Can you work these out from the model? Positions are in its coordinate system, mm. A direction names the side the tool comes from. Give positions to 0.01 mm unless a question says otherwise; leave off trailing zeros. Order: outer loops, then holes, each group sorted by start corner. A loop starts at its lowest first (then second) coordinate and runs counter-clockwise, first axis right, second up.
Item 1: I want a section at C-C, the plane y = -3.5. Write out the boundary of the cut face in (x, z).
Item 2: I'm going to push flat-ended pins straight in: pin 1 Ø3 at (x, y) = (7.5, 3.5) entering from +Z; pin 2 Ø1.5 at (x, y) = (3.5, 7.5) entering from -Z; pin 3 Ø1.5 at (x, z) = (2.5, 2.5) entering from +Y; pin 4 Ø1.5 at (y, z) = (-0.5, 4) entering from -X. Where does each tip first touch, or does it pass through?
Item 3: If we mould it in two halves opening along X, with no side actions, what happens to faces 1 (the cylindrical face through (-2.923, 6.391, 0.986)), 2 (the cylindrical face through (2.285, 3.584, 3.972)), 3 (the cylindrical face through (-3.77, -8.72, 0.99)), 4 (the flat face through (2.5, 2.5, 0))? For each: +X half, -X half, draft (parallel to the pull), parting line (faces both ways), or undercut.
Item 4: I want a section at D-D, the plane z = 1.75. Count the separate pieces of the cut face and the enclosed holes in it, then the cut area to 3 significant figures.
Item 5: I want a section at B-B, the plane y = 7.5. Write out the boundary of the cut face in (x, z), then the cut area to 3 significant figures.
Item 6: Which directions (+Z, -Z, +X, -X, +Y, -Y) give clear straight access to the entire face, cutting with the end or side of a thin tool? Please do faces 5 (the cylindrical face through (10, 3.2, 1)), 6 (the flat face through (5, 0, 2)).
Item 7: If I drill on line 1 along Y through (x, z) = (6.5, 1.9); line 2 along Z through (x, y) = (8.5, 4.75); line 3 along X through (y, z) = (-1.25, 4.7), over which ranges is the centre line in solid material (lowest first)?
Item 8: I want a section at A-A, the plane x = -7.75. Write out the boundary of the cut face in (y, z).
```python
from build123d import *

# Parameters (mm, degrees)
SKETCH5_R           = 10.5
SKETCH5_R_2         = 1.25
BOSS_EXTRUDE2_DEPTH = 2
SKETCH6_R           = 1.25
CUT_EXTRUDE2_DEPTH  = 2
SKETCH7_R           = 3
CUT_EXTRUDE3_DEPTH  = 1
SKETCH9_R           = 3
CUT_EXTRUDE5_DEPTH  = 5
SKETCH10_R          = 3
BOSS_EXTRUDE5_DEPTH = 2
SKETCH11_R          = 3.25
CUT_EXTRUDE6_DEPTH  = 2
SKETCH13_R          = 4.25
SKETCH13_R_2        = 3.25
BOSS_EXTRUDE6_DEPTH = 4


with BuildPart() as part:
    # Sketch5 → Boss-Extrude2 (new body)
    with BuildSketch(Plane.XY):
        Circle(SKETCH5_R)
        with Locations((0, 7.5)):
            Circle(SKETCH5_R_2, mode=Mode.SUBTRACT)
        with Locations((-3.5, 7.5)):
            Circle(SKETCH5_R_2, mode=Mode.SUBTRACT)
        with Locations((3.5, 7.5)):
            Circle(SKETCH5_R_2, mode=Mode.SUBTRACT)
        with Locations((-7.5, 0)):
            Circle(SKETCH5_R_2, mode=Mode.SUBTRACT)
        with Locations((-7.5, 3.5)):
            Circle(SKETCH5_R_2, mode=Mode.SUBTRACT)
        with Locations((-7.5, -3.5)):
            Circle(SKETCH5_R_2, mode=Mode.SUBTRACT)
        with Locations((0, -7.5)):
            Circle(SKETCH5_R_2, mode=Mode.SUBTRACT)
        with Locations((-3.5, -7.5)):
            Circle(SKETCH5_R_2, mode=Mode.SUBTRACT)
        with Locations((3.499264905, -7.428270452)):
            Circle(SKETCH5_R_2, mode=Mode.SUBTRACT)
        with Locations((7.5, 0)):
            Circle(SKETCH5_R_2, mode=Mode.SUBTRACT)
        with Locations((7.5, 3.5)):
            Circle(SKETCH5_R_2, mode=Mode.SUBTRACT)
        with Locations((7.5, -3.5)):
            Circle(SKETCH5_R_2, mode=Mode.SUBTRACT)
    extrude(amount=BOSS_EXTRUDE2_DEPTH)

    # Sketch6 → Cut-Extrude2 (cut)
    with BuildSketch(Plane(origin=(0, 0, 0), x_dir=(-1, 0, 0), z_dir=(0, 0, -1))):
        Circle(SKETCH6_R)
    extrude(amount=-CUT_EXTRUDE2_DEPTH, mode=Mode.SUBTRACT)

    # Sketch7 → Cut-Extrude3 (cut)
    with BuildSketch(Plane(origin=(0, 0, 0), x_dir=(-1, 0, 0), z_dir=(0, 0, -1))):
        Circle(SKETCH7_R)
    extrude(amount=-CUT_EXTRUDE3_DEPTH, mode=Mode.SUBTRACT)

    # Sketch9 → Cut-Extrude5 (cut)
    with BuildSketch(Plane(origin=(0, 0, 0), x_dir=(-1, 0, 0), z_dir=(0, 0, -1))):
        Circle(SKETCH9_R)
    extrude(amount=-CUT_EXTRUDE5_DEPTH, mode=Mode.SUBTRACT)

    # Sketch10 → Boss-Extrude5 (add)
    with BuildSketch(Plane(origin=(0, 0, 0), x_dir=(-1, 0, 0), z_dir=(0, 0, -1))):
        Circle(SKETCH10_R)
    extrude(amount=-BOSS_EXTRUDE5_DEPTH)

    # Sketch11 → Cut-Extrude6 (cut)
    with BuildSketch(Plane(origin=(0, 0, 0), x_dir=(-1, 0, 0), z_dir=(0, 0, -1))):
        Circle(SKETCH11_R)
    extrude(amount=-CUT_EXTRUDE6_DEPTH, mode=Mode.SUBTRACT)

    # Sketch13 → Boss-Extrude6 (add)
    with BuildSketch(Plane.XY.offset(2)):
        Circle(SKETCH13_R)
        with Locations(Location((0, 0, 0), (0, 0, 180))):
            Circle(SKETCH13_R_2, mode=Mode.SUBTRACT)
    extrude(amount=BOSS_EXTRUDE6_DEPTH)


solid = part.part
```
Results list:
1. outline: (-9.9, 0) - (-8.75, 0) - (-8.75, 2) - (-9.9, 2) - close; (-6.25, 0) - (6.25, 0) - (6.25, 2) - (2.41, 2) - (2.41, 6) - (-2.41, 6) - (-2.41, 2) - (-6.25, 2) - close; (8.75, 0) - (9.9, 0) - (9.9, 2) - (8.75, 2) - close
2. pin 1: stops at z = 2
2. pin 2: passes through
2. pin 3: stops at y = 10.32
2. pin 4: stops at x = -4.25
3. face 1: undercut
3. face 2: parting line
3. face 3: undercut
3. face 4: draft
4. separate pieces: 1
4. enclosed holes: 13
4. area: 254 mm2
5. outline: (-7.35, 0) - (-4.75, 0) - (-4.75, 2) - (-7.35, 2) - close; (-2.25, 0) - (-1.25, 0) - (-1.25, 2) - (-2.25, 2) - close; (1.25, 0) - (2.25, 0) - (2.25, 2) - (1.25, 2) - close; (4.75, 0) - (7.35, 0) - (7.35, 2) - (4.75, 2) - close
5. area: 14.4 mm2
6. face 5: +Z, -Z
6. face 6: +Z
7. line 1: y = -8.25 to -4.25, -2.75 to -0.75, 0.75 to 2.75, 4.25 to 8.25
7. line 2: z = 0 to 2
7. line 3: x = -4.06 to -3, 3 to 4.06
8. outline: (-7.08, 0) - (-4.72, 0) - (-4.72, 2) - (-7.08, 2) - close; (-2.28, 0) - (-1.22, 0) - (-1.22, 2) - (-2.28, 2) - close; (1.22, 0) - (2.28, 0) - (2.28, 2) - (1.22, 2) - close; (4.72, 0) - (7.08, 0) - (7.08, 2) - (4.72, 2) - close
